from build123d import *

# Parameters (mm, degrees)
ESQUISSE1_R                     = 2
BOSS_EXTRU_1_DEPTH              = 5
TROU_TARAUD_M3X0_51_D           = 2.5
TROU_TARAUD_M3X0_51_CSINK_D     = 3.05
TROU_TARAUD_M3X0_51_CSINK_ANGLE = 90
ENL_V_MAT_EXTRU_1_DEPTH         = 6
ENL_V_MAT_EXTRU_1_DEPTH_BACK    = 6


with BuildPart() as part:
    # Esquisse1 → Boss.-Extru.1 (new body, symmetric)
    with BuildSketch(Plane(origin=(0, 0, 0), x_dir=(1, 0, 0), z_dir=(0, 1, 0))):
        with BuildLine():
            Line((0, 5), (45, 5))
            ThreePointArc((45, 5), (50, 0), (45, -5))
            Line((45, -5), (0, -5))
            ThreePointArc((0, -5), (-5, 0), (0, 5))
        make_face()
        Circle(ESQUISSE1_R, mode=Mode.SUBTRACT)
    extrude(amount=BOSS_EXTRU_1_DEPTH, both=True)

    # Trou taraudé M3x0.51 (through all)
    with Locations(Plane(origin=(0, 5, 0), x_dir=(1, 0, 0), z_dir=(0, 1, 0))):
        with Locations((45, 0)):
            CounterSinkHole(TROU_TARAUD_M3X0_51_D / 2, TROU_TARAUD_M3X0_51_CSINK_D / 2, counter_sink_angle=TROU_TARAUD_M3X0_51_CSINK_ANGLE)

    # Esquisse4 → Enlèv. mat.-Extru.1 (cut, two sides)
    with BuildSketch(Plane.XY) as enl_v_mat_extru_1_sk:
        Polygon((35, 0), (50, 0), (50, -5), (30, -5), align=None)
    extrude(amount=ENL_V_MAT_EXTRU_1_DEPTH, mode=Mode.SUBTRACT)
    extrude(enl_v_mat_extru_1_sk.sketch, amount=-ENL_V_MAT_EXTRU_1_DEPTH_BACK, mode=Mode.SUBTRACT)


solid = part.part
Read the model definition and answer for the solid it produces. Units are mm, in the model's axes. A direction names the side the tool comes from. Give positions to 0.01 mm unless a question says otherwise; leave off trailing zeros. Write each loop counter-clockwise with the first axis right and the second up, starting at its lowest first coordinate (ties: lowest second). Pieces come first, ordered by that corner, then holes. Notation, with made-up numbers: (28, 42) - (53, 42) arc R22 ccw to (53, 68) - close; hole circle Ø9 at (77.5, 3). An arc over 180 degrees is marked (long way). Answer in a Markdown table with one row per item. Add a question column.
Item 1: A tool of negligible diameter and unlimited length cuts with its end or side. For faces 5 (the face through (23, 5, 0)), 6 (the face through (42, 0, 0)), from which of +Z, -Z, +X, -X, +Y, -Y can it reach the whole face along a straight path? Write none if from no direction.
Item 2: Section C-C, the plane y = -1.5 is taken. Write down the section's boundary in (x, z).
Item 3: Section A-A, the plane z = 0 is taken. Write down the section's boundary in (x, y) (3 decimals), and give its area (3 significant figures).
Item 4: Section D-D, the plane z = 3.75 is taken. Write down the section's boundary in (x, y), and give its area (3 significant figures).
Item 5: Flat-ended cylindrical pins translate along their axes: P1, Ø4, axis at y = -1, z = 3, coming from the -X side; P2, Ø4, axis at x = 45, z = 0, coming from the -Y side; P3, Ø4, axis at y = -0.5, z = -2.5, coming from the +X side. Find the tip coordinate at first contact, or state that the pin passes through.
Item 6: Find the intervals of material crossed by L1, parallel to Z at x = 0, y = -2.5; L2, parallel to X at y = 3.5, z = 0.75; L3, parallel to Z at x = 45, y = 3.2, in increasing order.
Item 7: Section B-B, the plane y = 2 is taken. Write down the section's boundary in (x, z).
Item 8: Determine the mould class of faces 1 (the face through (-5, 0, 0)), 2 (the face through (0, 0, 2)), 3 (the face through (46.25, 2.33, -0.05)), 4 (the face through (13, -5, 0)) for opening direction Z: pulls with the +Z half, pulls with the -Z half, needs draft (parallel to the pull), parting line crosses it, or undercut.
Recorded:
| question | item | result |
|---|---|---|
| 1 | face 5 | +Z, -Z, +X, -X, +Y |
| 1 | face 6 | +Z, -Z, +X, -Y |
| 2 | outline | (0, -5) - (33.5, -5) - (33.5, 5) - (0, 5) arc R5 ccw to start; hole circle Ø4 at (0, 0) |
| 3 | outline | (-5, -5) - (-2, -5) - (-2, 5) - (-5, 5) - close; (2, -5) - (30, -5) - (35, 0) - (43.75, 0) - (43.75, 4.725) - (43.475, 5) - (2, 5) - close; (46.25, 0) - (50, 0) - (50, 5) - (46.525, 5) - (46.25, 4.725) - close |
| 3 | area | 410 mm2 |
| 4 | outline | (-3.31, -5) - (30, -5) - (35, 0) - (48.31, 0) - (48.31, 5) - (-3.31, 5) - close |
| 4 | area | 437 mm2 |
| 5 | P1 | stops at x = -4.9 |
| 5 | P2 | stops at y = 0 |
| 5 | P3 | stops at x = 49.97 |
| 6 | L1 | z = -5 to -2, 2 to 5 |
| 6 | L2 | x = -4.94 to -1.85, 1.85 to 44, 46 to 49.94 |
| 6 | L3 | z = -5 to -1.25, 1.25 to 5 |
| 7 | outline | (0, -5) - (45, -5) arc R5 ccw to (45, 5) - (0, 5) arc R5 ccw to start; hole circle Ø4 at (0, 0); hole circle Ø2.5 at (45, 0) |
| 8 | face 1 | parting line crosses it |
| 8 | face 2 | undercut |
| 8 | face 3 | undercut |
| 8 | face 4 | needs draft |
